Part model, mm, in its own coordinate system. A direction names the side the tool comes from. Coordinates: 2 decimals unless noted, no trailing zeros. Order: outer loops, then holes, each group sorted by start corner. A loop starts at its lowest first (then second) coordinate and runs counter-clockwise, first axis right, second up. Notation, with made-up numbers: M 43,-22.75 L 49,-22.75 A25 ccw 49,13.25 Z; hole C -21,85 d9. An arc over 180 degrees is marked long. Answer in a Markdown table with one row per item. Add a question column.
from build123d import *

# Parameters (mm, degrees)
SKETCH1_W           = 101.6
SKETCH1_H           = 19.05
BOSS_EXTRUDE1_DEPTH = 12.7
SKETCH2_R           = 3.429
CUT_EXTRUDE1_DEPTH  = 56.72102386
SKETCH3_R           = 6.604
CUT_EXTRUDE4_DEPTH  = 6.985


with BuildPart() as part:
    # Sketch1 → Boss-Extrude1 (new body)
    with BuildSketch(Plane(origin=(0, 0, 0), x_dir=(1, 0, 0), z_dir=(0, 1, 0))):
        with Locations((0, 9.525)):
            Rectangle(SKETCH1_W, SKETCH1_H)
    extrude(amount=BOSS_EXTRUDE1_DEPTH)

    # Sketch2 → Cut-Extrude1 (cut, through all)
    with BuildSketch(Plane(origin=(0, 12.7, 0), x_dir=(1, 0, 0), z_dir=(0, 1, 0))):
        with Locations(Location((-38.1, 9.525, 0), (0, 0, 270))):
            Circle(SKETCH2_R)
        with Locations(Location((38.1, 9.525, 0), (0, 0, 270))):
            Circle(SKETCH2_R)
        with Locations(Location((-12.7, 9.525, 0), (0, 0, 270))):
            Circle(SKETCH2_R)
        with Locations(Location((12.7, 9.525, 0), (0, 0, 270))):
            Circle(SKETCH2_R)
    extrude(amount=-CUT_EXTRUDE1_DEPTH, mode=Mode.SUBTRACT)

    # Sketch3 → Cut-Extrude4 (cut)
    with BuildSketch(Plane(origin=(0, 0, 0), x_dir=(1, 0, 0), z_dir=(0, 1, 0))):
        with Locations(Location((-12.7, 9.525, 0), (0, 0, 270))):
            Circle(SKETCH3_R)
        with Locations(Location((12.7, 9.525, 0), (0, 0, 270))):
            Circle(SKETCH3_R)
    extrude(amount=CUT_EXTRUDE4_DEPTH, mode=Mode.SUBTRACT)


solid = part.part
(1) Slice it at C-C (z = -7). List the corners of the cut face in (x, y) (3 decimals).
(2) Drop flat-ended pins along their axis: P1, Ø9, axis at x = 12.7, z = -9.525, coming from the -Y side (3 decimals); P2, Ø4, axis at x = -38.1, z = -9.525, coming from the -Y side. Give the stop position or say it passes through.
(3) Slice it at D-D (x = -38.1). List the corners of the cut face in (y, z).
(4) 3-axis set-ups, long thin cutter, end or side, ignore diameter. For faces 1 (the cylindrical face through (38.25, 6.44, -12.95)), 2 (the flat face through (-16, 6.985, -7)): which of +Z, -Z, +X, -X, +Y, -Y reach the whole face in a straight line?
(5) Pull direction X, two halves, no side cores. Call faces 3 (the flat face through (-1, 6, 0)), 4 (the flat face through (-50.8, 6, -9)), 5 (the cylindrical face through (19.25, 3.44, -10.38)): pulls with the +X half, pulls with the -X half, needs draft (parallel to the pull), parting line crosses it, or undercut.
(6) Slice it at A-A (y = 2.75). List the corners of the cut face in (x, z) (3 decimals), and give its area (3 significant figures).
(7) Wall check: line 1 (X direction, y = 4.75, z = -9.5); line 2 (X direction, y = 6.75, z = -8.25); line 3 (X direction, y = 3.75, z = -13.25). Give the ranges that are in metal, low to high.
(8) Slice it at B-B (x = 12.7). List the corners of the cut face in (y, z) (3 decimals), and give its area (3 significant figures).
Computed:
| question | item | result |
|---|---|---|
| 1 | outline | M -50.8,0 L -40.42,0 L -40.42,12.7 L -50.8,12.7 Z; M -35.78,0 L -18.802,0 L -18.802,6.985 L -15.02,6.985 L -15.02,12.7 L -35.78,12.7 Z; M -10.38,6.985 L -6.598,6.985 L -6.598,0 L 6.598,0 L 6.598,6.985 L 10.38,6.985 L 10.38,12.7 L -10.38,12.7 Z; M 15.02,6.985 L 18.802,6.985 L 18.802,0 L 35.78,0 L 35.78,12.7 L 15.02,12.7 Z; M 40.42,0 L 50.8,0 L 50.8,12.7 L 40.42,12.7 Z |
| 2 | P1 | stops at y = 6.985 |
| 2 | P2 | passes through |
| 3 | outline | M 0,-19.05 L 12.7,-19.05 L 12.7,-12.95 L 0,-12.95 Z; M 0,-6.1 L 12.7,-6.1 L 12.7,0 L 0,0 Z |
| 4 | face 1 | +Y, -Y |
| 4 | face 2 | -Y |
| 5 | face 3 | needs draft |
| 5 | face 4 | pulls with the -X half |
| 5 | face 5 | undercut |
| 6 | outline | M -50.8,-19.05 L 50.8,-19.05 L 50.8,0 L -50.8,0 Z; hole C -38.1,-9.525 d6.858; hole C -12.7,-9.525 d13.208; hole C 12.7,-9.525 d13.208; hole C 38.1,-9.525 d6.858 |
| 6 | area | 1,590 mm^2 |
| 7 | line 1 | x = -50.8 to -41.53, -34.67 to -19.3, -6.1 to 6.1, 19.3 to 34.67, 41.53 to 50.8 |
| 7 | line 2 | x = -50.8 to -41.28, -34.92 to -19.18, -6.22 to 6.22, 19.18 to 34.92, 41.28 to 50.8 |
| 7 | line 3 | x = -50.8 to -18.15, -7.25 to 7.25, 18.15 to 50.8 |
| 8 | outline | M 0,-19.05 L 12.7,-19.05 L 12.7,-12.954 L 6.985,-12.954 L 6.985,-16.129 L 0,-16.129 Z; M 0,-2.921 L 6.985,-2.921 L 6.985,-6.096 L 12.7,-6.096 L 12.7,0 L 0,0 Z |
| 8 | area | 110 mm^2 |
